```python
from build123d import *

# Parameters (mm, degrees)
F0_R     = 1.75
F0_R_2   = 1.5
F1_DEPTH = 4
F2_R     = 2.6
F2_R_2   = 1.75
F3_DEPTH = 0.2
F4_R     = 0.24999


# Not quite as in the source:
# - a fillet or chamfer that OpenCascade refuses, or shapes differently, is made with other operations: its cross-section is extruded or revolved along the edge and cut away or added
# - a fillet or chamfer is up to 0.001 mm smaller than in the source, because OpenCascade refuses the exact size


with BuildPart() as f1:
    # F0 (on Front) → F1 (new body)
    with BuildSketch(Plane.XZ):
        Circle(F0_R)
        Circle(F0_R_2, mode=Mode.SUBTRACT)
    extrude(amount=F1_DEPTH)

    # F2 (on Front) → F3 (join)
    with BuildSketch(Plane.XZ):
        Circle(F2_R)
        Circle(F2_R_2, mode=Mode.SUBTRACT)
    extrude(amount=F3_DEPTH)

    # F4 (radius 0.25 in the source; OpenCascade refuses exactly that, so slightly less here)
    f4_edges = [f1.edges().sort_by_distance(p)[0] for p in [
        (-1.75, -4, 0),
    ]]
    fillet(f4_edges, radius=F4_R)

    # F5: fillet of radius 0.5 on 2 edges, made by hand

    # F5_s1 → F5_t2 (revolve, cut)
    with BuildSketch(Plane.XY):
        with BuildLine():
            ThreePointArc((2.6, -0.2), (2.4236067977, -0.0527864045), (2.2, 0))
            Line((2.2, 0), (2.6, 0))
            Line((2.6, 0), (2.6, -0.2))
        make_face()
    revolve(axis=Axis((0, 0, 0), (0, -1, 0)), mode=Mode.SUBTRACT)

    # F5_s3 → F5_t4 (revolve, cut)
    with BuildSketch(Plane.XY):
        with BuildLine():
            ThreePointArc((1.5, -0.5), (1.6464466094, -0.1464466094), (2, 0))
            Line((2, 0), (1.5, 0))
            Line((1.5, 0), (1.5, -0.5))
        make_face()
    revolve(axis=Axis((0, 0, 0), (0, -1, 0)), mode=Mode.SUBTRACT)


solid = f1.part
```
The model under review builds one solid part; all positions refer to its coordinate system, in mm. Round coordinates to 2 decimals unless told otherwise and drop trailing zeros. Loops run counter-clockwise (first coordinate to the right, second up) from the corner with the lowest first, then second, coordinate; pieces in that order, holes last. Notation, with made-up numbers: (34, 11) - (93, 11) arc R24 ccw to (93, 30) - close; hole circle Ø11 at (-25.75, 48.25). An arc over 180 degrees is marked (long way). Use a Markdown table: item, result. Add a question column.
Q1. Insertion check: pin 1 Ø1 at (y, z) = (-1.5, 0.5) entering from +X. The pin has a flat end and moves straight along its axis. Give the tip position at first contact, or say it passes through.
Q2. The part is to be moulded in two halves that separate along X. For faces 1 (the face through (-1.5, -2.23, 0.07)), 2 (the face through (2, -0.2, -1)), 3 (the face through (1.617, -1.95, -0.67)), say which applies: pulls with the +X half, pulls with the -X half, needs draft (parallel to the pull), parting line crosses it, or undercut.
Q3. For probe 1 along Z at (x, y) = (0, -2.8); probe 2 along Z at (x, y) = (1.25, -0.4); probe 3 along X at (y, z) = (-1.7, 0.15), list the stretches that pass through material, from the lowest coordinate up.
Q4. Add section C-C (y = -3.3). State the section outline as (x, z) points.
Worked answers:
| question | item | result |
|---|---|---|
| 1 | pin 1 | x = 1.75 |
| 2 | face 1 | undercut |
| 2 | face 2 | needs draft |
| 2 | face 3 | parting line crosses it |
| 3 | probe 1 | -1.75 to -1.5, 1.5 to 1.75 |
| 3 | probe 2 | -1.22 to -0.85, 0.85 to 1.22 |
| 3 | probe 3 | -1.74 to -1.49, 1.49 to 1.74 |
| 4 | outline | circle Ø3.5 at (0, 0); hole circle Ø3 at (0, 0) |
